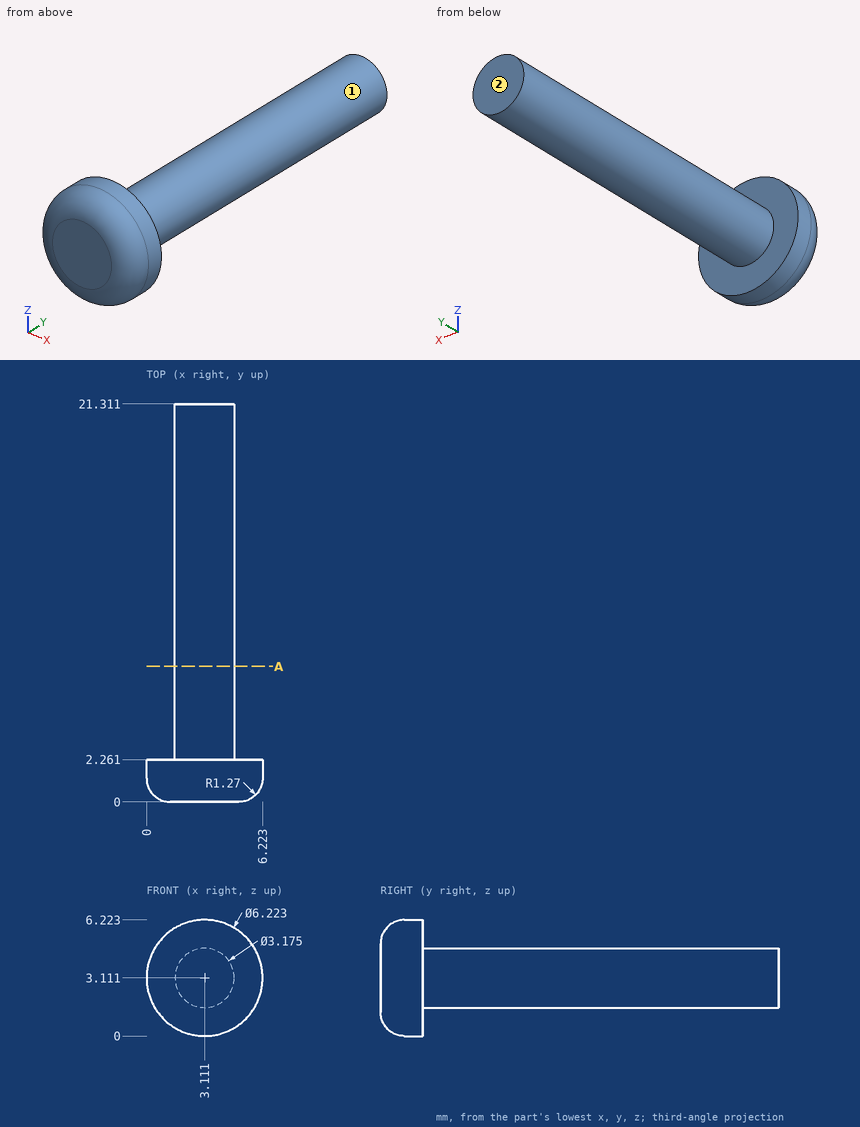
Geometry check sheet. Reference: drawing and pictorial views, mm from the part's lowest x, y, z. A direction names the side the tool comes from. Give positions to 0.01 mm unless a question says otherwise; leave off trailing zeros. Write each loop counter-clockwise with the first axis right and the second up, starting at its lowest first coordinate (ties: lowest second). Pieces come first, ordered by that corner, then holes. Notation, with made-up numbers: M 20.5,12.25 L 32.5,12.25 A33 cw 32.5,43.25 Z; hole C 22,65 d4. An arc over 180 degrees is marked long. Answer as CSV lines item,"result". Start each with the question number.
Q1. Section check A-A, the plane y = 7.25. Record the cut outline in (x, z) (1 decimal).
Q2. Go/stop test with flat-tipped pins: pin 1 (3 mm diameter, centred on y = 11, z = 4, fed in from +X); pin 2 (3 mm diameter, centred on x = 5, z = 2.5, fed in from +Y). Record where each tip stops, or that it passes through.
Q3. Material ranges on L1, parallel to X at y = 11.75, z = 2.5 (1 decimal); L2, parallel to Y at x = 3.25, z = 1; L3, parallel to Z at x = 3.25, y = 1, recorded low to high.
Q4. Tool access check on the marked faces 1 and 2. Record the directions out of +Z, -Z, +X, -X, +Y, -Y that give a thin tool (end or side, any length) a straight path to the whole face; none if there is none.
Geometry says:
1,outline,"C 3.1,3.1 d3.2"
2,pin 1,"x = 4.7"
2,pin 2,"y = 21.31"
3,L1,"1.6 to 4.6"
3,L2,"0.03 to 2.26"
3,L3,"0.03 to 6.19"
4,face 1,"+Y"
4,face 2,"+Z, -Z, +X, -X, +Y"
